```python
from build123d import *

# Parameters (mm, degrees)
BOSS_EXTRUDE1_DEPTH = 3750
SCALE1_SCALE        = 0.001
BOSS_EXTRUDE2_DEPTH = 3.75
SKETCH7_R           = 6
BOSS_EXTRUDE4_DEPTH = 8.5
CUT_EXTRUDE2_DEPTH  = 7.5
SKETCH9_R           = 4
CUT_EXTRUDE3_DEPTH  = 4.75


# Read off the part's stored shape, not the designer's step: Imported1
with BuildPart() as part:
    # Sketch1 → Boss-Extrude1 (new body)
    with BuildSketch(Plane.XY):
        Polygon((-1706.06803894, 17555.067062378), (-569.962084293, 15778.41758728), (-1006.988286972, 15208.873748779), (-3063.715457916, 15425.035476685), (-3388.391971588, 14641.19720459), (-1831.166863441, 13219.130516052), (-2105.892896652, 12555.883407593), (-4148.485660553, 12232.358932495), (-4259.226799011, 11391.19720459), (-2387.004852295, 10420.625686646), (-2480.708837509, 9708.873748779), (-4369.967937469, 8867.712020874), (-4259.226799011, 8026.550292969), (-2199.596881866, 7573.616504669), (-2105.892896652, 6861.864089966), (-3713.068246841, 5560.388088226), (-3388.391971588, 4776.549816132), (-1281.714439392, 4872.121334076), (-1006.988286972, 4208.873748779), (-2222.553491592, 2535.776615143), (-1706.06803894, 1862.679600716), (304.090321064, 2500.242710114), (741.116523743, 1930.699110031), (0, 0), (673.097014427, -516.485512257), (2449.747562408, 619.62044239), (3019.291162491, 182.594239712), (2803.129196167, -1874.132990837), (3586.967229843, -2198.8093853), (5009.034156799, -641.584277153), (5672.281742096, -916.310429573), (5995.805263519, -2958.903074265), (6836.967468262, -3069.644212723), (7807.538509369, -1197.422385216), (8519.290924072, -1291.12637043), (9360.452651978, -3180.385351181), (10201.615333557, -3069.644212723), (10654.54864502, -1010.014414787), (11366.300582886, -916.310429573), (12667.777061462, -2523.485660553), (13451.615333557, -2198.8093853), (13356.043815613, -92.131927609), (14019.290924072, 182.594239712), (15692.388534546, -1032.971024513), (16365.48614502, -516.485512257), (15727.922439575, 1493.672847748), (16297.466278076, 1930.699110031), (18228.164672852, 1189.582586288), (18744.649887085, 1862.679600716), (17608.543395996, 3639.330148697), (18045.570373535, 4208.873748779), (20102.296829224, 3992.711782455), (20426.973342896, 4776.549816132), (18869.749069214, 6198.616504669), (19144.47593689, 6861.864089966), (21187.06703186, 7185.388088226), (21297.80960083, 8026.550292969), (19425.586700439, 8997.120857239), (19519.290924072, 9708.873748779), (21408.550262451, 10550.035476685), (21297.80960083, 11391.19720459), (19238.178253174, 11844.130516052), (19144.47593689, 12555.883407593), (20751.649856567, 13857.358932495), (20426.973342896, 14641.19720459), (18320.297241211, 14545.625686646), (18045.570373535, 15208.873748779), (19261.135101318, 16881.971359253), (18744.649887085, 17555.067062378), (16734.491348267, 16917.505264282), (16297.466278076, 17487.049102783), (17038.581848145, 19417.747497559), (16365.48614502, 19934.232711792), (14588.834762573, 18798.126220703), (14019.290924072, 19235.153198242), (14235.452651978, 21291.879653931), (13451.615333557, 21616.556167603), (12029.54864502, 20059.331893921), (11366.300582886, 20334.056854248), (11042.777061462, 22376.649856567), (10201.615333557, 22487.392425537), (9231.043815613, 20615.169525146), (8519.290924072, 20708.873748779), (7678.129196167, 22598.133087158), (6836.967468262, 22487.392425537), (6384.034156799, 20427.761077881), (5672.281742096, 20334.056854248), (4370.805263519, 21941.232681274), (3586.967229843, 21616.556167603), (3682.538747787, 19509.880065918), (3019.291162491, 19235.153198242), (1346.194028854, 20450.717926025), (673.097014427, 19934.232711792), (1310.660123825, 17924.074172974), (741.116523743, 17487.049102783), (-1189.582586288, 18228.164672852), align=None)
    extrude(amount=BOSS_EXTRUDE1_DEPTH)


with BuildPart() as part_1:
    # Scale1: scaled about (8519.290960158, 9708.873493624, 1875)
    add(part.part.scale(SCALE1_SCALE).moved(Location((8510.771669198, 9699.16462013, 1873.125))))


with BuildPart() as body_2:
    # Sketch4 → Boss-Extrude2 (new body)
    with BuildSketch(Plane.XY.offset(1876.875)):
        Polygon((8482.082875407, 9717.46612407), (8483.52052795, 9719.007817674), (8484.291694952, 9718.650324381), (8484.044201424, 9716.556903507), (8484.601498068, 9716.182821727), (8486.44519641, 9717.204800407), (8487.06814831, 9716.626500372), (8486.185865351, 9714.712018515), (8486.600288328, 9714.184031467), (8488.669558431, 9714.586256829), (8489.083316356, 9713.843758089), (8487.65260797, 9712.295618071), (8487.883590672, 9711.665408806), (8489.975877959, 9711.40850823), (8490.139940401, 9710.574491734), (8488.300854292, 9709.544236288), (8488.325786523, 9708.873494079), (8490.236283338, 9707.982614784), (8490.134590722, 9707.138719878), (8488.067149452, 9706.727197584), (8487.883590672, 9706.081579353), (8489.425284275, 9704.64392681), (8489.067790982, 9703.872759808), (8486.974370108, 9704.120253336), (8486.600288328, 9703.562956692), (8487.622267008, 9701.71925835), (8487.043966973, 9701.09630645), (8485.129485116, 9701.978589409), (8484.601498068, 9701.564166432), (8485.00372343, 9699.494896329), (8484.26122469, 9699.081138404), (8482.713084672, 9700.51184679), (8482.082875407, 9700.280864088), (8481.825974831, 9698.188576801), (8480.991958335, 9698.024514359), (8479.961702889, 9699.863600468), (8479.29096068, 9699.838668237), (8478.400081385, 9697.928171422), (8477.556186479, 9698.029864038), (8477.144664185, 9700.097305308), (8476.499045954, 9700.280864088), (8475.061393411, 9698.739170485), (8474.290226409, 9699.096663778), (8474.537719937, 9701.190084652), (8473.980423293, 9701.564166432), (8472.136724951, 9700.542187752), (8471.513773051, 9701.120487787), (8472.39605601, 9703.034969644), (8471.981633033, 9703.562956692), (8469.91236293, 9703.16073133), (8469.498605005, 9703.90323007), (8470.929313391, 9705.451370088), (8470.698330689, 9706.081579353), (8468.606043402, 9706.338479929), (8468.44198096, 9707.172496425), (8470.281067069, 9708.202751871), (8470.256134838, 9708.873494079), (8468.345638023, 9709.764373375), (8468.447330639, 9710.608268281), (8470.514771909, 9711.019790575), (8470.698330689, 9711.665408806), (8469.156637086, 9713.103061349), (8469.514130379, 9713.874228351), (8471.607551253, 9713.626734823), (8471.981633033, 9714.184031467), (8470.959654353, 9716.027729809), (8471.537954388, 9716.650681709), (8473.452436245, 9715.76839875), (8473.980423293, 9716.182821727), (8473.578197931, 9718.25209183), (8474.320696671, 9718.665849755), (8475.868836689, 9717.235141369), (8476.499045954, 9717.46612407), (8476.75594653, 9719.558411358), (8477.589963026, 9719.7224738), (8478.620218472, 9717.883387691), (8479.29096068, 9717.908319922), (8480.181839976, 9719.818816737), (8481.025734882, 9719.71712412), (8481.437257176, 9717.649682851), align=None)
    extrude(amount=BOSS_EXTRUDE2_DEPTH)

    # Sketch7 → Boss-Extrude4 (add)
    with BuildSketch(Plane.XY.offset(1880.625)):
        with Locations(Location((8479.29096068, 9708.873494079, 0), (0, 0, 180))):
            Circle(SKETCH7_R)
    extrude(amount=BOSS_EXTRUDE4_DEPTH)

    # Sketch8 → Cut-Extrude2 (cut)
    with BuildSketch(Plane.XY.offset(1889.125)):
        with BuildLine():
            Line((8476.579872338, 9710.573494079), (8482.002049023, 9710.573494079))
            ThreePointArc((8482.002049023, 9710.573494079), (8479.29096068, 9705.673494079), (8476.579872338, 9710.573494079))
        make_face()
    extrude(amount=-CUT_EXTRUDE2_DEPTH, mode=Mode.SUBTRACT)

    # Sketch9 → Cut-Extrude3 (cut)
    with BuildSketch(Plane(origin=(0, 0, 1876.875), x_dir=(-1, 0, 0), z_dir=(0, 0, -1))):
        with Locations((-8479.29096068, 9708.873494079)):
            Circle(SKETCH9_R)
    extrude(amount=-CUT_EXTRUDE3_DEPTH, mode=Mode.SUBTRACT)


solid = body_2.part
```
Could you check a few things on this model? Use its own coordinates, in mm. A direction names the side the tool comes from. Coordinates: 2 decimals unless noted, no trailing zeros. Write each loop counter-clockwise with the first axis right and the second up, starting at its lowest first coordinate (ties: lowest second). Pieces come first, ordered by that corner, then holes. Notation, with made-up numbers: (80, 61) -> (121, 61) arc R22 cw to (121, 85) -> close; hole circle Ø1 at (9, 78). An arc over 180 degrees is marked (long way). Write item = value, one per line. Start each with the question number.
(1) I want a section at A-A (y = 9710.25). Please give me the cut outline in (x, z) (3 decimals), plus the area to 3 significant figures.
(2) I need wall thicknesses on line 1 (Y direction, x = 8487, z = 1878.5); line 2 (X direction, y = 9718.75, z = 1879.25); line 3 (Z direction, x = 8486.75, y = 9705.5) (3 decimals). Which ranges of each line are inside material? Lowest first, please. Write a range as [from, to].
(3) Will these pins go through, and if not, where does the flat tip stop? pin 1 (1.6 mm diameter, centred on x = 8479, z = 1885.5, fed in from -Y); pin 2 (1.5 mm diameter, centred on x = 8477, z = 1883.5, fed in from -Y); pin 3 (1 mm diameter, centred on x = 8484.5, z = 1879, fed in from -Y).
(4) I want a section at C-C (z = 1888.5). Please give me the cut outline in (x, y).
(5) Which directions (+Z, -Z, +X, -X, +Y, -Y) give clear straight access to the entire face, cutting with the end or side of a thin tool? Please do faces 4 (the face through (8478.852, 9698.897, 1878.724)), 5 (the face through (8486.63, 9715.68, 1878.72)), 6 (the face through (8470.55, 9713.75, 1878.72)), 7 (the face through (8479, 9711, 1881.625)), 8 (the face through (8469.667, 9706.208, 1878.724)).
(6) We'd pull the mould along Y, two halves only. Please class faces 1 (the face through (8488, 9704, 1879)), 2 (the face through (8481.23, 9718.7, 1878.72)), 3 (the face through (8468.525, 9706.75, 1878.724)): released by +Y, released by -Y, zero draft, split by the parting line, or undercut.
(7) I want a section at B-B (x = 8480.5). Please give me the cut outline in (y, z) (1 decimal), plus the area to 3 significant figures.
Result set:
q1.outline = (8468.404, 1876.875) -> (8475.535, 1876.875) -> (8475.535, 1881.625) -> (8476.402, 1881.625) -> (8476.402, 1889.125) -> (8473.451, 1889.125) -> (8473.451, 1880.625) -> (8468.404, 1880.625) -> close; (8482.18, 1881.625) -> (8483.047, 1881.625) -> (8483.047, 1876.875) -> (8489.561, 1876.875) -> (8489.561, 1880.625) -> (8485.131, 1880.625) -> (8485.131, 1889.125) -> (8482.18, 1889.125) -> close
q1.area = 99.6 mm2
q2.line_1 = [9701.12, 9702.84], [9704.12, 9714.26], [9716.48, 9716.69]
q2.line_2 = [8476.66, 8478.13], [8479.68, 8481.22], [8483.28, 8484.08]
q2.line_3 = [1876.875, 1880.625]
q3.pin_1 = 9702.87
q3.pin_2 = 9703.07
q3.pin_3 = 9699.08
q4.outline = circle Ø12 at (8479.29, 9708.87); hole (8476.58, 9710.57) arc R3.2 ccw (long way) to (8482, 9710.57) -> close
q5.face_4 = +Z, -Z, -Y
q5.face_5 = +Z, -Z, +X
q5.face_6 = +Z, -Z
q5.face_7 = -Z
q5.face_8 = +Z, -Z, -X
q6.face_1 = undercut
q6.face_2 = released by +Y
q6.face_3 = released by -Y
q7.outline = (9698.9, 1876.9) -> (9705.1, 1876.9) -> (9705.1, 1881.6) -> (9705.9, 1881.6) -> (9705.9, 1889.1) -> (9703, 1889.1) -> (9703, 1880.6) -> (9698.9, 1880.6) -> close; (9710.6, 1881.6) -> (9712.7, 1881.6) -> (9712.7, 1876.9) -> (9719.8, 1876.9) -> (9719.8, 1880.6) -> (9714.8, 1880.6) -> (9714.8, 1889.1) -> (9710.6, 1889.1) -> close
q7.area = 107 mm2
